The listing builds one solid part. Answer for the finished solid, in the listing's coordinates (mm). Coordinates: 2 decimals unless noted, no trailing zeros. Loops run counter-clockwise (first coordinate to the right, second up) from the corner with the lowest first, then second, coordinate; pieces in that order, holes last. Notation, with made-up numbers: (7, 26) -> (25, 26) arc R33 ccw to (25, 60) -> close; hole circle Ø7 at (9.5, 28.5). An arc over 180 degrees is marked (long way). Answer in a Markdown table with one row per item.
```python
from build123d import *

# Parameters (mm, degrees)
F0_R     = 6.35
F1_DEPTH = 19.05


with BuildPart() as f1:
    # F0 (on Front) → F1 (new body)
    with BuildSketch(Plane.XZ):
        with BuildLine():
            ThreePointArc((6.35, -50.8), (4.490128, -46.309872), (0, -44.45))
            ThreePointArc((0, -44.45), (-4.490128, -55.290128), (6.35, -50.8))
        make_face()
        with BuildLine():
            ThreePointArc((-12.7, 50.8), (-23.358147, 23.358147), (-50.8, 12.7))
            ThreePointArc((-50.8, 12.7), (-63.5, 0), (-50.8, -12.7))
            ThreePointArc((-50.8, -12.7), (-23.358147, -23.358147), (-12.7, -50.8))
            ThreePointArc((-12.7, -50.8), (0, -63.5), (12.7, -50.8))
            ThreePointArc((12.7, -50.8), (23.358147, -23.358147), (50.8, -12.7))
            ThreePointArc((50.8, -12.7), (63.5, 0), (50.8, 12.7))
            ThreePointArc((50.8, 12.7), (23.358147, 23.358147), (12.7, 50.8))
            ThreePointArc((12.7, 50.8), (0, 63.5), (-12.7, 50.8))
        make_face()
        with BuildLine():
            ThreePointArc((6.35, -50.8), (-4.490128, -55.290128), (0, -44.45))
            ThreePointArc((0, -44.45), (4.490128, -46.309872), (6.35, -50.8))
        make_face(mode=Mode.SUBTRACT)
        with Locations((-50.8, 0)):
            Circle(F0_R, mode=Mode.SUBTRACT)
        with BuildLine():
            ThreePointArc((12.7, 0), (8.980256, -8.980256), (0, -12.7))
            ThreePointArc((0, -12.7), (-8.980256, -8.980256), (-12.7, 0))
            ThreePointArc((-12.7, 0), (0, 12.7), (12.7, 0))
        make_face(mode=Mode.SUBTRACT)
        with Locations((50.8, 0)):
            Circle(F0_R, mode=Mode.SUBTRACT)
        with Locations((0, 50.8)):
            Circle(F0_R, mode=Mode.SUBTRACT)
    extrude(amount=F1_DEPTH)


solid = f1.part
```
Item 1: Find the intervals of material crossed by probe 1 along X at (y, z) = (-14.5, 50.5); probe 2 along Z at (x, y) = (-50.8, -3.75); probe 3 along X at (y, z) = (-7.25, -11), in increasing order.
Findings below:
| item | result |
|---|---|
| probe 1 | x = -12.69 to -6.34, 6.34 to 12.69 |
| probe 2 | z = -12.7 to -6.35, 6.35 to 12.7 |
| probe 3 | x = -57.15 to -6.35, 6.35 to 57.15 |
Item 2: A cutting plane is placed at B-B, the plane x = 32.5. Determine the outline of the cut face in (y, z).
Findings below:
| item | result |
|---|---|
| outline | (-19.05, -16.69) -> (0, -16.69) -> (0, 16.69) -> (-19.05, 16.69) -> close |
Item 3: Flat-ended cylindrical pins translate along their axes: pin 1 Ø4 at (x, y) = (9.5, -3.5) entering from -Z; pin 2 Ø3 at (x, y) = (-8, -13) entering from -Z; pin 3 Ø4 at (y, z) = (-2, 48.5) entering from +X. Find the tip coordinate at first contact, or state that the pin passes through.
Findings below:
| item | result |
|---|---|
| pin 1 | stops at z = -61.05 |
| pin 2 | stops at z = -61.71 |
| pin 3 | stops at x = 12.76 |
Item 4: A cutting plane is placed at C-C, the plane z = -19. Determine the outline of the cut face in (x, y).
Findings below:
| item | result |
|---|---|
| outline | (-28.62, -19.05) -> (28.62, -19.05) -> (28.62, 0) -> (-28.62, 0) -> close |
Item 5: A cutting plane is placed at A-A, the plane y = -4. Count the separate pieces of the cut face and the enclosed holes in it, plus the area to 3 significant figures.
Findings below:
| item | result |
|---|---|
| separate pieces | 1 |
| enclosed holes | 5 |
| area | 5,650 mm2 |
Item 6: Determine the mould class of faces 1 (the face through (9.1, -19.05, -9.1)), 2 (the face through (63.497, -9.392, -0.279)), 3 (the face through (-0.279, -9.392, -63.497)), 4 (the face through (56.857, -9.392, 1.907)) for opening direction Z: +Z half, -Z half, draft (parallel to the pull), parting line (faces both ways), or undercut.
Findings below:
| item | result |
|---|---|
| face 1 | draft |
| face 2 | parting line |
| face 3 | -Z half |
| face 4 | undercut |
